Autodesk Inventor part; units mm, degrees
ref_plane "YZ Plane" through (0, 0, 0) normal (1, 0, 0) x (0, 1, 0)
ref_plane "XZ Plane" through (0, 0, 0) normal (0, 1, 0) x (-1, 0, 0)
ref_plane "XY Plane" through (0, 0, 0) normal (0, 0, 1) x (1, 0, 0)
sketch "Sketch1" plane through (0, 0, 0) normal (0, 1, 0) x (-1, 0, 0)
  line L0 (-35, -60) -> (35, -60)
  line L1 (35, -60) -> (35, 60)
  line L2 (35, 60) -> (-35, 60)
  line L3 (-35, 60) -> (-35, -60)
  line L4 (-35, -60) -> (35, 60) construction
  line L5 (35, -60) -> (-35, 60) construction
  point P0 (0, 0)
  dimension "d0" = 70
  dimension "d1" = 120
extrude "Extrusion1" add sketch "Sketch1" along normal blind 3
sketch "Sketch2" plane through (0, 3, 0) normal (0, 1, 0) x (1, 0, 0)
  line L0 (35, -60) -> (32, -60)
  line L1 (32, -60) -> (32, -50)
  line L2 (32, -50) -> (35, -50)
  line L3 (35, -50) -> (35, -60)
  line L4 (35, -5) -> (32, -5)
  line L5 (32, -5) -> (32, 5)
  line L6 (32, 5) -> (35, 5)
  line L7 (35, 5) -> (35, -5)
  line L8 (35, 50) -> (32, 50)
  line L9 (32, 50) -> (32, 60)
  line L10 (32, 60) -> (35, 60)
  line L11 (35, 60) -> (35, 50)
  line L12 (35, -60) -> (35, 60)
  point P0 (0, 0)
  point P1 (35, 0)
  dimension "d4" = 3
  dimension "d5" = 10
  dimension "d6" = 3
  dimension "d7" = 10
  dimension "d8" = 10
extrude "Extrusion2" cut sketch "Sketch2" against normal through all
sketch "Sketch3" plane through (0, 0, 0) normal (0, -1, 0) x (1, 0, 0)
  line L0 (32, -60) -> (-35, -60)
  line L1 (3.5, 63) -> (-6.5, 63)
  line L2 (-6.5, 63) -> (-6.5, 60)
  line L3 (-6.5, 60) -> (3.5, 60)
  line L4 (3.5, 60) -> (3.5, 63)
  line L5 (3.5, -60) -> (-6.5, -60)
  line L6 (-6.5, -60) -> (-6.5, -63)
  line L7 (-6.5, -63) -> (3.5, -63)
  line L8 (3.5, -63) -> (3.5, -60)
  line L9 (-35, -60) -> (-35, 60)
  line L10 (-35, 60) -> (-25, 60)
  line L11 (-25, 60) -> (-25, 63)
  line L12 (-25, 63) -> (-35, 63)
  line L13 (-35, 63) -> (-35, 60)
  line L14 (-35, -60) -> (-25, -60)
  line L15 (-25, -60) -> (-25, -63)
  line L16 (-25, -63) -> (-35, -63)
  line L17 (-35, -63) -> (-35, -60)
  point P0 (0, 0)
  point P1 (32, 60)
  point P2 (-1.5, 60)
  point P3 (-1.5, -60)
  dimension "d15" = 10
  dimension "d16" = 3
  dimension "d17" = 10
  dimension "d18" = 3
  dimension "d21" = 10
  dimension "d22" = 10
extrude "Extrusion3" add sketch "Sketch3" against normal blind 3 contours L8 L7 L6 L0 | L4 L3 L2 L1
sketch "Sketch4" plane through (0, 0, 0) normal (0, -1, 0) x (1, 0, 0)
  line L0 (-38, -36.5) -> (-35, -36.5)
  line L1 (-35, -36.5) -> (-35, -26.5)
  line L2 (-35, -26.5) -> (-38, -26.5)
  line L3 (-38, -26.5) -> (-38, -36.5)
  line L4 (-38, 26.5) -> (-35, 26.5)
  line L5 (-35, 26.5) -> (-35, 36.5)
  line L6 (-35, 36.5) -> (-38, 36.5)
  line L7 (-38, 36.5) -> (-38, 26.5)
  line L8 (-35, -60) -> (-35, 60)
  point P0 (0, 0)
  point P1 (-35, -31.5)
  point P2 (-35, -63)
  point P3 (-35, 63)
  point P4 (-35, 31.5)
  point P5 (-35, 0)
  point P6 (-35, 0)
  dimension "d23" = 3
  dimension "d24" = 10
  dimension "d25" = 3
  dimension "d26" = 10
  dimension "d27" = 126
  dimension "d28" = 31.5
  dimension "d29" = 31.5
extrude "Extrusion4" add sketch "Sketch4" against normal blind 3
sketch "Sketch5" plane through (0, 3, 0) normal (0, 1, 0) x (1, 0, 0)
  line L0 (35, -50) -> (32, -50)
  line L1 (32, -50) -> (32, -60)
  line L2 (32, -60) -> (3.5, -60)
  line L3 (3.5, -60) -> (3.5, -63)
  line L4 (3.5, -63) -> (-6.5, -63)
  line L5 (-6.5, -63) -> (-6.5, -60)
  line L6 (-6.5, -60) -> (-35, -60)
  line L7 (-35, -60) -> (-35, -36.5)
  line L8 (-35, -36.5) -> (-38, -36.5)
  line L9 (-38, -36.5) -> (-38, -26.5)
  line L10 (-38, -26.5) -> (-35, -26.5)
  line L11 (-35, -26.5) -> (-35, 26.5)
  line L12 (-35, 26.5) -> (-38, 26.5)
  line L13 (-38, 26.5) -> (-38, 36.5)
  line L14 (-38, 36.5) -> (-35, 36.5)
  line L15 (-35, 36.5) -> (-35, 60)
  line L16 (-35, 60) -> (-6.5, 60)
  line L17 (-6.5, 60) -> (-6.5, 63)
  line L18 (-6.5, 63) -> (3.5, 63)
  line L19 (3.5, 63) -> (3.5, 60)
  line L20 (3.5, 60) -> (32, 60)
  line L21 (32, 60) -> (32, 50)
  line L22 (32, 50) -> (35, 50)
  line L23 (35, 50) -> (35, 5)
  line L24 (35, 5) -> (32, 5)
  line L25 (32, 5) -> (32, -5)
  line L26 (32, -5) -> (35, -5)
  line L27 (35, -5) -> (35, -50)
  point P0 (0, 0)
properties part number "Bottom"
Work out the finished part from the listing and answer in its coordinate system (mm). A direction names the side the tool comes from. Give positions to 0.01 mm unless a question says otherwise; leave off trailing zeros. Order: outer loops, then holes, each group sorted by start corner. A loop starts at its lowest first (then second) coordinate and runs counter-clockwise, first axis right, second up. Notation, with made-up numbers: (-40, 84.5) - (-2, 84.5) arc R23 ccw to (-2, 123.5) - close; hole circle Ø2 at (88.25, 30). An arc over 180 degrees is marked (long way). Answer as CSV lines item,"result". Start each with the question number.
Q1. For faces 1 (the face through (34, 2, -50)), 2 (the face through (-21, 1, 60)), 3 (the face through (-37, 1, -36.5)), 4 (the face through (18, 1, 60)), 5 (the face through (-35, 1, 0)), determine the directions among +Z, -Z, +X, -X, +Y, -Y from which every point of the face is accessible in a straight line to the end or side of a thin tool.
Q2. The mould has two halves that part along Z. Classify faces 6 (the face through (-38, 1, -31)), 7 (the face through (33, 2, -5)), 8 (the face through (-21, 1, -60)): +Z half, -Z half, draft (parallel to the pull), parting line (faces both ways), or undercut.
Q3. Given pin 1 Ø1.5 at (x, y) = (11.5, 2) entering from +Z; pin 2 Ø1.5 at (x, y) = (-37, 2) entering from -Z; pin 3 Ø0.9 at (y, z) = (1, -45) entering from -X, each flat-ended and moving along its own axis, determine where each tip first touches the part or whether it passes through.
Q4. Find the intervals of material crossed by L1, parallel to Z at x = 31.5, y = 1.35; L2, parallel to X at y = 1.5, z = -8.5; L3, parallel to X at y = 2.65, z = 2, in increasing order. Write a range as [from, to].
Q5. The part is cut by section C-C (x = -8). Write down the section's boundary in (y, z).
Q6. The part is cut by section B-B (z = 2.5). Write down the section's boundary in (x, y).
Q7. The part is cut by section A-A (y = 0.75). Write down the section's boundary in (x, z).
Check result:
1,face 1,"-Z, +X, +Y, -Y"
1,face 2,"+Z, -X, +Y, -Y"
1,face 3,"-Z, -X, +Y, -Y"
1,face 4,"+Z, +X, +Y, -Y"
1,face 5,"-X, +Y, -Y"
2,face 6,"draft"
2,face 7,"undercut"
2,face 8,"-Z half"
3,pin 1,"stops at z = 60"
3,pin 2,"stops at z = -36.5"
3,pin 3,"stops at x = -35"
4,L1,"z = [-60, 60]"
4,L2,"x = [-35, 35]"
4,L3,"x = [-35, 32]"
5,outline,"(0, -60) - (3, -60) - (3, 60) - (0, 60) - close"
6,outline,"(-35, 0) - (32, 0) - (32, 3) - (-35, 3) - close"
7,outline,"(-38, -36.5) - (-35, -36.5) - (-35, -60) - (-6.5, -60) - (-6.5, -63) - (3.5, -63) - (3.5, -60) - (32, -60) - (32, -50) - (35, -50) - (35, -5) - (32, -5) - (32, 5) - (35, 5) - (35, 50) - (32, 50) - (32, 60) - (3.5, 60) - (3.5, 63) - (-6.5, 63) - (-6.5, 60) - (-35, 60) - (-35, 36.5) - (-38, 36.5) - (-38, 26.5) - (-35, 26.5) - (-35, -26.5) - (-38, -26.5) - close"
